Read the model definition and answer for the solid it produces. Units are mm, in the model's axes. A direction names the side the tool comes from. Coordinates: 2 decimals unless noted, no trailing zeros. Write each loop counter-clockwise with the first axis right and the second up, starting at its lowest first coordinate (ties: lowest second). Pieces come first, ordered by that corner, then holes.
(1) Given pin 1 (1 mm diameter, centred on y = 6.5, z = 4, fed in from -X); pin 2 (1.5 mm diameter, centred on x = 3, y = -5.5, fed in from +Z), each flat-ended and moving along its own axis, determine where each tip first touches the part or whether it passes through.
(2) The part is cut by section A-A, the plane x = 0. Determine the outline of the cut face in (y, z).
(3) Which of the six approach directions +Z, -Z, +X, -X, +Y, -Y give full straight-line access (tool end or side, diameter ignored) to faces 1 (the flat face through (0, 0, 0)), 2 (the cylindrical face through (-6, 0, 2))?
(4) Straight lines are drawn through the part: line 1 along Z through (x, y) = (-2.75, -2.75); line 2 along Z through (x, y) = (5.25, -5.5); line 3 along X through (y, z) = (-0.5, 5.2). For each, find the intervals that lie inside material, in ascending order.
(5) The part is cut by section C-C, the plane z = 4.1. Determine the outline of the cut face in (x, y).
```python
from build123d import *

# Parameters (mm, degrees)
F0_R     = 10
F0_R_2   = 6
F1_DEPTH = 1.5
F0_R_3   = 3.5
F2_DEPTH = 2.5
F3_DEPTH = 5.5
F4_SIZE  = 1


with BuildPart() as f1:
    # F0 (on Top) → F1 (new body)
    with BuildSketch(Plane.XY):
        Circle(F0_R)
        Circle(F0_R_2, mode=Mode.SUBTRACT)
    extrude(amount=F1_DEPTH)

    # F0 (on Top) → F2 (join)
    with BuildSketch(Plane.XY):
        Circle(F0_R_2)
        Circle(F0_R_3, mode=Mode.SUBTRACT)
    extrude(amount=F2_DEPTH)

    # F0 (on Top) → F3 (join)
    with BuildSketch(Plane.XY):
        Circle(F0_R_3)
    extrude(amount=F3_DEPTH)

    # F4
    f4_edges = [f1.edges().sort_by_distance(p)[0] for p in [
        (-10, 0, 0),
    ]]
    chamfer(f4_edges, length=F4_SIZE)


solid = f1.part
```
Computed:
1. pin 1: passes through
1. pin 2: stops at z = 2.5
2. outline: (-10, 1) - (-9, 0) - (9, 0) - (10, 1) - (10, 1.5) - (6, 1.5) - (6, 2.5) - (3.5, 2.5) - (3.5, 5.5) - (-3.5, 5.5) - (-3.5, 2.5) - (-6, 2.5) - (-6, 1.5) - (-10, 1.5) - close
3. face 1: -Z, +X, -X, +Y, -Y
3. face 2: +Z
4. line 1: z = 0 to 2.5
4. line 2: z = 0 to 1.5
4. line 3: x = -3.46 to 3.46
5. outline: circle Ø7 at (0, 0)
